For this review, take the finished solid that the model builds, in its own axes (mm). Face numbers are marked on the shaded views. A direction names the side the tool comes from. Give positions to 0.01 mm unless a question says otherwise; leave off trailing zeros. Write each loop counter-clockwise with the first axis right and the second up, starting at its lowest first coordinate (ties: lowest second). Pieces come first, ordered by that corner, then holes.
from build123d import *

# Parameters (mm, degrees)
BOSS_EXTRUDE1_DEPTH = 15.24
BOSS_EXTRUDE2_DEPTH = 15.24
SKETCH6_W           = 37.211
SKETCH6_H           = 30.861
CUT_EXTRUDE1_DEPTH  = 5.2705
SKETCH7_W           = 37.211
SKETCH7_H           = 4.699
BOSS_EXTRUDE3_DEPTH = 2.159


with BuildPart() as part:
    # Sketch3 → Boss-Extrude1 (new body)
    with BuildSketch(Plane(origin=(0, 0, 0), x_dir=(1, 0, 0), z_dir=(0, 1, 0))):
        with BuildLine():
            Line((2.54, 0), (10.16, 0))
            Line((10.16, 0), (12.7, 0))
            Line((12.7, 0), (12.7, 2.54))
            Line((12.7, 2.54), (12.7, 36.83))
            Line((12.7, 36.83), (12.7, 39.37))
            Line((12.7, 39.37), (10.16, 39.37))
            Line((10.16, 39.37), (2.54, 39.37))
            ThreePointArc((2.54, 39.37), (0.743948776, 38.626051224), (0, 36.83))
            Line((0, 36.83), (0, 2.54))
            ThreePointArc((0, 2.54), (0.743948776, 0.743948776), (2.54, 0))
        make_face()
        with BuildLine():
            Line((5.08, 6.604), (7.62, 6.604))
            ThreePointArc((7.62, 6.604), (8.518025612, 6.975974388), (8.89, 7.874))
            Line((8.89, 7.874), (8.89, 31.496))
            ThreePointArc((8.89, 31.496), (8.518025612, 32.394025612), (7.62, 32.766))
            Line((7.62, 32.766), (5.08, 32.766))
            ThreePointArc((5.08, 32.766), (4.181974388, 32.394025612), (3.81, 31.496))
            Line((3.81, 31.496), (3.81, 7.874))
            ThreePointArc((3.81, 7.874), (4.181974388, 6.975974388), (5.08, 6.604))
        make_face(mode=Mode.SUBTRACT)
    extrude(amount=BOSS_EXTRUDE1_DEPTH)

    # Sketch4 → Boss-Extrude2 (add)
    with BuildSketch(Plane(origin=(0, 0, 0), x_dir=(1, 0, 0), z_dir=(0, 1, 0))):
        with BuildLine():
            Line((12.7, 39.37), (13.335, 39.37))
            ThreePointArc((13.335, 39.37), (21.6535, 31.0515), (29.972, 39.37))
            Line((29.972, 39.37), (49.911, 39.37))
            Line((49.911, 39.37), (49.911, 0))
            Line((49.911, 0), (29.972, 0))
            ThreePointArc((29.972, 0), (21.6535, 8.3185), (13.335, 0))
            Line((13.335, 0), (12.7, 0))
            Line((12.7, 0), (12.7, 39.37))
        make_face()
    extrude(amount=BOSS_EXTRUDE2_DEPTH)

    # Sketch6 → Cut-Extrude1 (cut, symmetric)
    with BuildSketch(Plane(origin=(0, 7.62, 0), x_dir=(1, 0, 0), z_dir=(0, 1, 0))):
        with Locations((31.3055, 19.685)):
            Rectangle(SKETCH6_W, SKETCH6_H)
    extrude(amount=CUT_EXTRUDE1_DEPTH, both=True, mode=Mode.SUBTRACT)

    # Sketch7 → Boss-Extrude3 (add)
    with BuildSketch(Plane(origin=(0, 2.3495, 0), x_dir=(1, 0, 0), z_dir=(0, 1, 0))):
        with Locations((31.3055, 19.685)):
            Rectangle(SKETCH7_W, SKETCH7_H)
    boss_extrude3 = extrude(amount=BOSS_EXTRUDE3_DEPTH)

    # Mirror1: Boss-Extrude3 across plane
    add(boss_extrude3.mirror(Plane.ZX.offset(7.62)))


solid = part.part
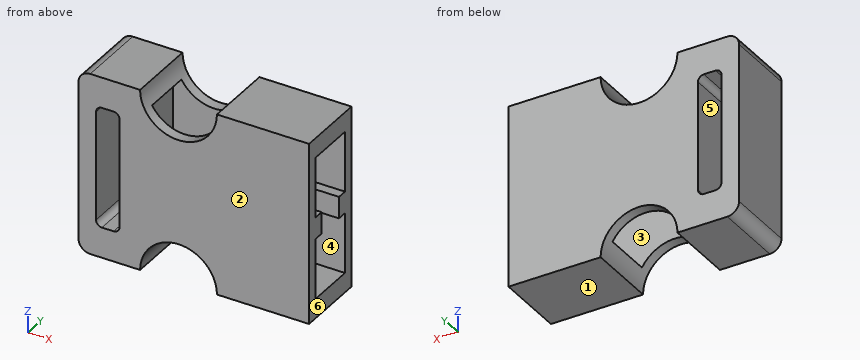
(1) Tool access review of the marked faces 4, 5 and 6: name each direction out of +Z, -Z, +X, -X, +Y, -Y from which nothing blocks a thin tool from reaching the whole face with its end or side.
(2) Clearance check with flat-ended pins moving along their axes: pin 1 Ø5.5 at (x, y) = (42.5, 6) entering from +Z; pin 2 Ø6 at (x, y) = (26, 7) entering from +Z; pin 3 Ø4 at (x, y) = (17.5, 5) entering from +Z; pin 4 Ø1.1 at (x, y) = (26, 3) entering from -Z. State where each tip first meets the part, or that it passes through.
(3) The part is to be moulded in two halves that separate along Y. For the marked faces 1, 2 and 3, say which applies: +Y half, -Y half, draft (parallel to the pull), parting line (faces both ways), or undercut.
(4) We need section A-A (y = 7.75). Write out the cut boundary in (x, z) (1 decimal), and give its area (3 significant figures).
(5) We need section D-D (x = 33.5). Write out the cut boundary in (y, z), and give its area (3 significant figures).
(6) We need section B-B (x = 7). Write out the cut boundary in (y, z).
(7) For L1, parallel to Z at x = 35.5, y = 12.75; L2, parallel to X at y = 14.75, z = -24.5; L3, parallel to Y at x = 21, z = -28.5, list the stretches that pass through material, from the lowest coordinate up.
(8) We need section C-C (z = -27). Write out the cut boundary in (x, y).
The answers:
1. face 4: +X
1. face 5: +Y, -Y
1. face 6: +Z, -Z, +X, +Y, -Y
2. pin 1: stops at z = 0
2. pin 2: stops at z = -3.9
2. pin 3: stops at z = -17.34
2. pin 4: stops at z = -22.03
3. face 1: draft
3. face 2: -Y half
3. face 3: undercut
4. outline: (0, -36.8) arc R2.5 ccw to (2.5, -39.4) - (13.3, -39.4) arc R8.3 cw to (14.5, -35.1) - (12.7, -35.1) - (12.7, -4.3) - (14.5, -4.3) arc R8.3 cw to (13.3, 0) - (2.5, 0) arc R2.5 ccw to (0, -2.5) - close; (28.8, -35.1) arc R8.3 cw to (30, -39.4) - (49.9, -39.4) - (49.9, -35.1) - close; (28.8, -4.3) - (49.9, -4.3) - (49.9, 0) - (30, 0) arc R8.3 cw to start; hole (3.8, -31.5) arc R1.3 ccw to (5.1, -32.8) - (7.6, -32.8) arc R1.3 ccw to (8.9, -31.5) - (8.9, -7.9) arc R1.3 ccw to (7.6, -6.6) - (5.1, -6.6) arc R1.3 ccw to (3.8, -7.9) - close
4. area: 547 mm2
5. outline: (0, -39.37) - (15.24, -39.37) - (15.24, 0) - (0, 0) - close; hole (2.35, -35.12) - (12.89, -35.12) - (12.89, -22.03) - (10.73, -22.03) - (10.73, -17.34) - (12.89, -17.34) - (12.89, -4.25) - (2.35, -4.25) - (2.35, -17.34) - (4.51, -17.34) - (4.51, -22.03) - (2.35, -22.03) - close
5. area: 295 mm2
6. outline: (0, -39.37) - (15.24, -39.37) - (15.24, -32.77) - (0, -32.77) - close; (0, -6.6) - (15.24, -6.6) - (15.24, 0) - (0, 0) - close
7. L1: z = -39.37 to -35.12, -22.03 to -17.34, -4.25 to 0
7. L2: x = 0 to 3.81, 8.89 to 49.91
7. L3: y = 0 to 2.35, 12.89 to 15.24
8. outline: (0, 0) - (3.81, 0) - (3.81, 15.24) - (0, 15.24) - close; (8.89, 0) - (49.91, 0) - (49.91, 2.35) - (12.7, 2.35) - (12.7, 12.89) - (49.91, 12.89) - (49.91, 15.24) - (8.89, 15.24) - close
